Part model, mm, in its own coordinate system. A direction names the side the tool comes from. Give positions to 0.01 mm unless a question says otherwise; leave off trailing zeros. Order: outer loops, then holes, each group sorted by start corner. A loop starts at its lowest first (then second) coordinate and runs counter-clockwise, first axis right, second up. Notation, with made-up numbers: M 50.5,-1.75 L 103.5,-1.75 A30 ccw 103.5,20.25 Z; hole C -13,84.5 d8. An arc over 180 degrees is marked long. Return JSON: item names as keys, results as strings.
from build123d import *

# Parameters (mm, degrees)
BOSS_EXTRUDE1_DEPTH = 4
CUT_EXTRUDE1_DEPTH  = 4
SKETCH3_R           = 0.8
CUT_EXTRUDE2_DEPTH  = 4
SKETCH4_R           = 0.8
CUT_EXTRUDE3_DEPTH  = 4
BOSS_EXTRUDE2_DEPTH = 14.5
CUT_EXTRUDE4_DEPTH  = 4
SKETCH15_W          = 32.370090848
SKETCH15_H          = 10.5
CUT_EXTRUDE6_DEPTH  = 4
CIRPATTERN1_COUNT   = 6
BOSS_EXTRUDE3_DEPTH = 21
SKETCH19_W          = 32.370090848
SKETCH19_H          = 17
CUT_EXTRUDE7_DEPTH  = 4
CIRPATTERN2_COUNT   = 6
BOSS_EXTRUDE4_DEPTH = 17
CIRPATTERN3_COUNT   = 6


with BuildPart() as part:
    # Sketch1 → Boss-Extrude1 (new body)
    with BuildSketch(Plane(origin=(0, 0, 0), x_dir=(1, 0, 0), z_dir=(0, 1, 0))):
        Polygon((0, 60), (-51.961524227, 30), (-51.961524227, -30), (0, -60), (51.961524227, -30), (51.961524227, 30), align=None)
    extrude(amount=BOSS_EXTRUDE1_DEPTH)

    # Sketch2 → Cut-Extrude1 (cut)
    with BuildSketch(Plane(origin=(0, 4, 0), x_dir=(1, 0, 0), z_dir=(0, 1, 0))):
        Polygon((38.961524227, 0), (38.961524227, 7.2), (51.961524227, 7.2), (51.961524227, -17.8), (38.961524227, -17.8), align=None)
        Polygon((19.480762114, 33.741669751), (13.245379206, 37.341669751), (19.745379206, 48.6), (41.396014301, 36.1), (34.896014301, 24.841669751), align=None)
        Polygon((19.480762114, -33.741669751), (25.716145021, -30.141669751), (32.216145021, -41.4), (10.565509926, -53.9), (4.065509926, -42.641669751), align=None)
        Polygon((-19.480762114, -33.741669751), (-13.245379206, -37.341669751), (-19.745379206, -48.6), (-41.396014301, -36.1), (-34.896014301, -24.841669751), align=None)
        Polygon((-38.961524227, 0), (-38.961524227, -7.2), (-51.961524227, -7.2), (-51.961524227, 17.8), (-38.961524227, 17.8), align=None)
        Polygon((-19.480762114, 33.741669751), (-25.716145021, 30.141669751), (-32.216145021, 41.4), (-10.565509926, 53.9), (-4.065509926, 42.641669751), align=None)
    extrude(amount=-CUT_EXTRUDE1_DEPTH, mode=Mode.SUBTRACT)

    # Sketch3 → Cut-Extrude2 (cut)
    with BuildSketch(Plane(origin=(0, 4, 0), x_dir=(1, 0, 0), z_dir=(0, 1, 0))):
        with Locations(Location((15.196341101, 43.720834875, 0), (0, 0, 270))):
            Circle(SKETCH3_R)
        with Locations(Location((39.445052407, 29.720834875, 0), (0, 0, 90))):
            Circle(SKETCH3_R)
        with Locations(Location((45.461524227, 8.7, 0), (0, 0, 270))):
            Circle(SKETCH3_R)
        with Locations(Location((45.461524227, -19.3, 0), (0, 0, 90))):
            Circle(SKETCH3_R)
        with Locations(Location((30.265183126, -35.020834875, 0), (0, 0, 270))):
            Circle(SKETCH3_R)
        with Locations(Location((6.016471821, -49.020834875, 0), (0, 0, 90))):
            Circle(SKETCH3_R)
        with Locations(Location((-15.196341101, -43.720834875, 0), (0, 0, 270))):
            Circle(SKETCH3_R)
        with Locations(Location((-39.445052407, -29.720834875, 0), (0, 0, 90))):
            Circle(SKETCH3_R)
        with Locations(Location((-45.461524227, -8.7, 0), (0, 0, 270))):
            Circle(SKETCH3_R)
        with Locations(Location((-45.461524227, 19.3, 0), (0, 0, 90))):
            Circle(SKETCH3_R)
        with Locations(Location((-30.265183126, 35.020834875, 0), (0, 0, 270))):
            Circle(SKETCH3_R)
        with Locations(Location((-6.01647182, 49.020834875, 0), (0, 0, 90))):
            Circle(SKETCH3_R)
    extrude(amount=-CUT_EXTRUDE2_DEPTH, mode=Mode.SUBTRACT)

    # Sketch4 → Cut-Extrude3 (cut)
    with BuildSketch(Plane(origin=(0, 4, 0), x_dir=(1, 0, 0), z_dir=(0, 1, 0))):
        with Locations(Location((36.961524227, -5.3, 0), (0, 0, 270))):
            Circle(SKETCH4_R)
        with Locations(Location((13.890827473, -34.659618943, 0), (0, 0, 270))):
            Circle(SKETCH4_R)
        with Locations(Location((-36.961524227, 5.3, 0), (0, 0, 270))):
            Circle(SKETCH4_R)
        with Locations(Location((-13.890827473, 34.659618943, 0), (0, 0, 270))):
            Circle(SKETCH4_R)
    extrude(amount=-CUT_EXTRUDE3_DEPTH, mode=Mode.SUBTRACT)

    # Sketch12 → Boss-Extrude2 (add)
    with BuildSketch(Plane.XZ):
        Polygon((34.961524227, 0), (34.961524227, 20.185045424), (17.480762114, 30.277568136), (0, 40.370090848), (-17.480762114, 30.277568136), (-34.961524227, 20.185045424), (-34.961524227, 0), (-34.961524227, -20.185045424), (-17.480762114, -30.277568136), (0, -40.370090848), (17.480762114, -30.277568136), (34.961524227, -20.185045424), align=None)
        Polygon((-30.961524227, 0), (-30.961524227, -17.875644347), (-15.480762114, -26.813466521), (0, -35.751288694), (15.480762114, -26.813466521), (30.961524227, -17.875644347), (30.961524227, 0), (30.961524227, 17.875644347), (15.480762114, 26.813466521), (0, 35.751288694), (-15.480762114, 26.813466521), (-30.961524227, 17.875644347), align=None, mode=Mode.SUBTRACT)
    extrude(amount=BOSS_EXTRUDE2_DEPTH)

    # Sketch14 → Cut-Extrude4 (cut)
    with BuildSketch(Plane.XZ):
        Polygon((0, -35.751288694), (30.961524227, -17.875644347), (30.961524227, 17.875644347), (0, 35.751288694), (-30.961524227, 17.875644347), (-30.961524227, -17.875644347), align=None)
    extrude(amount=-CUT_EXTRUDE4_DEPTH, mode=Mode.SUBTRACT)

    # Sketch15 → Cut-Extrude6 (cut)
    with BuildSketch(Plane.ZY.offset(34.961524227)):
        with Locations((0, -5.25)):
            Rectangle(SKETCH15_W, SKETCH15_H)
    cut_extrude6 = extrude(amount=-CUT_EXTRUDE6_DEPTH, mode=Mode.SUBTRACT)

    # CirPattern1: Cut-Extrude6 ×6 about axis
    cirpattern1_axis = Axis((0, 0, 0), (0, 1, 0))
    for i in range(1, CIRPATTERN1_COUNT):
        add(cut_extrude6.rotate(cirpattern1_axis, i * 360 / CIRPATTERN1_COUNT), mode=Mode.SUBTRACT)

    # Sketch17 → Boss-Extrude3 (add)
    with BuildSketch(Plane(origin=(0, 4, 0), x_dir=(1, 0, 0), z_dir=(0, 1, 0))):
        Polygon((-34.961524227, 0), (-34.961524227, -20.185045424), (-17.480762114, -30.277568136), (0, -40.370090848), (17.480762114, -30.277568136), (34.961524227, -20.185045424), (34.961524227, 0), (34.961524227, 20.185045424), (17.480762114, 30.277568136), (0, 40.370090848), (-17.480762114, 30.277568136), (-34.961524227, 20.185045424), align=None)
        Polygon((30.961524227, -17.875644347), (30.961524227, 0), (30.961524227, 17.875644347), (15.480762114, 26.813466521), (0, 35.751288694), (-15.480762114, 26.813466521), (-30.961524227, 17.875644347), (-30.961524227, 0), (-30.961524227, -17.875644347), (-15.480762114, -26.813466521), (0, -35.751288694), (15.480762114, -26.813466521), align=None, mode=Mode.SUBTRACT)
    extrude(amount=BOSS_EXTRUDE3_DEPTH)

    # Sketch19 → Cut-Extrude7 (cut)
    with BuildSketch(Plane(origin=(17.480762114, 0, 30.277568136), x_dir=(0.8660254037844386, 0, -0.5000000000000001), z_dir=(0.5000000000000001, 0, 0.8660254037844386))):
        with Locations((0, 12.5)):
            Rectangle(SKETCH19_W, SKETCH19_H)
    cut_extrude7 = extrude(amount=-CUT_EXTRUDE7_DEPTH, mode=Mode.SUBTRACT)

    # CirPattern2: Cut-Extrude7 ×6 about axis
    cirpattern2_axis = Axis((0, 0, 0), (0, 1, 0))
    for i in range(1, CIRPATTERN2_COUNT):
        add(cut_extrude7.rotate(cirpattern2_axis, i * 360 / CIRPATTERN2_COUNT), mode=Mode.SUBTRACT)

    # Sketch23 → Boss-Extrude4 (add)
    with BuildSketch(Plane.XZ.offset(-21)):
        Polygon((15.315698604, 31.527568136), (19.645825623, 29.027568136), (17.645825623, 25.563466521), (13.315698604, 28.063466521), align=None)
    boss_extrude4 = extrude(amount=BOSS_EXTRUDE4_DEPTH)

    # CirPattern3: Boss-Extrude4 ×6 about axis
    cirpattern3_axis = Axis((0, 0, 0), (0, 1, 0))
    for i in range(1, CIRPATTERN3_COUNT):
        add(boss_extrude4.rotate(cirpattern3_axis, i * 360 / CIRPATTERN3_COUNT))


solid = part.part
Q1. 3-axis set-ups, long thin cutter, end or side, ignore diameter. For faces 3 (the flat face through (-19, 0, 26)), 4 (the flat face through (-2.5, 12.4, -36.7)), 5 (the flat face through (2.5, 12.4, 36.7)), 6 (the flat face through (-33, 12, 16.185)), 7 (the flat face through (7.36, 2.03, 48.35)): which of +Z, -Z, +X, -X, +Y, -Y reach the whole face in a straight line?
Established:
{"face 3": "none", "face 4": "-X", "face 5": "+X", "face 6": "+X, -X", "face 7": "+X, +Y, -Y"}
Q2. Band-saw the part on B-B (y = 12). Give the number of separate pieces and of enclosed holes in the cut face, then the cut area to 3 significant figures.
Established:
{"separate pieces": "12", "enclosed holes": "0", "area": "257 mm²"}
Q3. Band-saw the part on C-C (x = -23.5). Give the cut face in (y, z).
Established:
{"outline": "M -14.5,-26.8 L -10.5,-26.8 L -10.5,-22.18 L -14.5,-22.18 Z; M -14.5,22.18 L -10.5,22.18 L -10.5,26.8 L -14.5,26.8 Z; M 0,-31.42 L 4,-31.42 L 4,-22.18 L 0,-22.18 Z; M 0,22.18 L 4,22.18 L 4,31.42 L 0,31.42 Z; M 21,-26.8 L 25,-26.8 L 25,-22.18 L 21,-22.18 Z; M 21,22.18 L 25,22.18 L 25,26.8 L 21,26.8 Z"}
Q4. Band-saw the part on A-A (x = 8.5). Give the cut face in (y, z).
Established:
{"outline": "M -14.5,-35.46 L -10.5,-35.46 L -10.5,-30.84 L -14.5,-30.84 Z; M -14.5,30.84 L -10.5,30.84 L -10.5,35.46 L -14.5,35.46 Z; M 0,-55.09 L 4,-55.09 L 4,-30.84 L 0,-30.84 Z; M 0,30.84 L 4,30.84 L 4,40.08 L 0,40.08 Z; M 0,50.32 L 4,50.32 L 4,55.09 L 0,55.09 Z; M 21,-35.46 L 25,-35.46 L 25,-30.84 L 21,-30.84 Z; M 21,30.84 L 25,30.84 L 25,35.46 L 21,35.46 Z"}
Q5. Probe line 1 along X through (y, z) = (2.6, -5.3); line 2 along X through (y, z) = (21.5, -4.5); line 3 along X through (y, z) = (1, -8). List the from-to ranges inside material, lowest first.
Established:
{"line 1": "x = -38.96 to -37.76, -36.16 to -30.96, 30.96 to 38.96", "line 2": "x = -34.96 to -30.96, 30.96 to 34.96", "line 3": "x = -38.96 to -30.96, 30.96 to 45.07, 45.85 to 51.96"}
Q6. Two-plate mould, pull along Y, no slides. Class faces 1 (the flat face through (-51.962, 2, -24)), 2 (the flat face through (30.511, -5.323, 20.477)): +Y half, -Y half, draft (parallel to the pull), parting line (faces both ways), or undercut.
Established:
{"face 1": "draft", "face 2": "undercut"}
Q7. Pin check, flat tips, straight feed: pin 1 (4 mm diameter, centred on y = 10.5, z = 1, fed in from -X); pin 2 (10 mm diameter, centred on x = -1.5, y = 4, fed in from +Z); pin 3 (4.5 mm diameter, centred on x = 32, y = -5, fed in from +Z); pin 4 (1.5 mm diameter, centred on y = 12.5, z = -35.5, fed in from -X). Stop position of each tip, or through.
Established:
{"pin 1": "stops at x = -34.96", "pin 2": "stops at z = 60", "pin 3": "stops at z = 22.19", "pin 4": "stops at x = -2.24"}
